```python
from build123d import *

# Parameters (mm, degrees)
SKETCH1_R           = 3
BOSS_EXTRUDE2_DEPTH = 12
SKETCH3_W           = 14.680148962
SKETCH3_H           = 3.5
CUT_EXTRUDE1_DEPTH  = 214.215717845
CUT_EXTRUDE4_DEPTH  = 6


with BuildPart() as part:
    # Sketch1 → Boss-Extrude2 (new body)
    with BuildSketch(Plane(origin=(0, 0, 0), x_dir=(1, 0, 0), z_dir=(0, 1, 0))):
        with BuildLine():
            ThreePointArc((49.32216584, -188.806160656), (56.59547157, -193.17640364), (60.965714553, -185.903097909))
            Line((60.965714554, -185.903097909), (16.76676248, -8.63078365))
            ThreePointArc((16.76676248, -8.63078365), (15.305067103, -5.385940236), (12.79956958, -2.858482163))
            Line((12.79956958, -2.858482163), (-5.735764363, 10.120098388))
            ThreePointArc((-5.735764363, 10.120098388), (-8.870108332, 13.694132698), (-10, 18.311618831))
            Line((-10, 18.311618831), (-10, 50.355948326))
            ThreePointArc((-10, 50.355948326), (-10.073223305, 50.532725021), (-10.25, 50.605948326))
            Line((-10.25, 50.605948326), (-11.322967039, 50.605948326))
            ThreePointArc((-11.322967039, 50.605948326), (-11.883595848, 50.434015556), (-12.251443729, 49.977339002))
            Line((-12.251443729, 49.977339002), (-13.876153382, 45.915564871))
            ThreePointArc((-13.876153382, 45.915564871), (-13.982191925, 45.601023533), (-14.052832331, 45.276692901))
            Line((-14.052832331, 45.276692901), (-19.445744306, 11.667622342))
            ThreePointArc((-19.445744306, 11.667622342), (-19.325125521, 8.055028023), (-17.928078586, 4.721314409))
            Line((-17.928078586, 4.721314409), (12.801336755, -42.329115693))
            Line((12.801336755, -42.329115693), (49.322165839, -188.806160656))
        make_face()
        with BuildLine():
            Line((53.747443969, -171.212996829), (57.618194299, -186.737728449))
            ThreePointArc((57.618194299, -186.737728449), (55.76084103, -189.828883385), (52.669686095, -187.971530117))
            Line((52.669686095, -187.971530117), (48.798935765, -172.446798496))
            ThreePointArc((48.798935765, -172.446798496), (50.656289033, -169.355643561), (53.747443969, -171.212996829))
        make_face(mode=Mode.SUBTRACT)
        with Locations(Location((0, 0, 0), (0, 0, 270))):
            Circle(SKETCH1_R, mode=Mode.SUBTRACT)
    extrude(amount=BOSS_EXTRUDE2_DEPTH)

    # Sketch3 → Cut-Extrude1 (cut, through all)
    with BuildSketch(Plane(origin=(-20.818600927, 0, -3.11186707), x_dir=(-0.15843335293481708, 0, 0.9873696737685596), z_dir=(-0.9873696737685597, 0, -0.1584333529348171))):
        Polygon((-42.704193729, 0), (-8.890997144, 0), (-22.384342691, 3.5), (-42.704193729, 3.5), align=None)
        Polygon((-22.384342691, 8.5), (-8.890997144, 12), (-42.704193729, 12), (-42.704193729, 8.5), align=None)
        with Locations((-50.04426821, 10.25)):
            Rectangle(SKETCH3_W, SKETCH3_H)
        with Locations((-50.04426821, 1.75)):
            Rectangle(SKETCH3_W, SKETCH3_H)
    extrude(amount=-CUT_EXTRUDE1_DEPTH, mode=Mode.SUBTRACT)

    # Sketch4 → Cut-Extrude4 (cut)
    with BuildSketch(Plane(origin=(0, 12, 0), x_dir=(1, 0, 0), z_dir=(0, 1, 0))):
        Polygon((-4.95077941, 9.570446006), (-17.928078586, 4.721314409), (8.620757021, -35.928145405), (10.712205441, -18.154940656), (16.76676248, -8.63078365), (17.432158169, -2.976226879), align=None)
    extrude(amount=-CUT_EXTRUDE4_DEPTH, mode=Mode.SUBTRACT)


solid = part.part
```
Design review of the part built by this model. Coordinates are the model's own, in mm. A direction names the side the tool comes from. Coordinates: 2 decimals unless noted, no trailing zeros. Order: outer loops, then holes, each group sorted by start corner. A loop starts at its lowest first (then second) coordinate and runs counter-clockwise, first axis right, second up.
1) Take a section at A-A, the plane x = 0. Give the boundary of the cut face in (y, z).
2) Clearance check with flat-ended pins moving along their axes: pin 1 (8 mm diameter, centred on x = -15, z = -39, fed in from -Y); pin 2 (2 mm diameter, centred on x = -14.5, z = -32, fed in from +Y); pin 3 (3 mm diameter, centred on y = 8, z = 94.5, fed in from +X). State where each tip first meets the part, or that it passes through.
3) Take a section at C-C, the plane z = 29. Give the boundary of the cut face in (x, y), and give its area (3 significant figures).
4) Wall thickness on line 1 along Z through (x, y) = (0, 3.95); line 2 along X through (y, z) = (6.5, 182.5); line 3 along Z through (x, y) = (0.5, 2): over which ranges is each line inside the solid? List them lowest first.
5) Take a section at B-B, the plane z = 0. Give the boundary of the cut face in (x, y), and give its area (3 significant figures).
6) Take a section at D-D, the plane x = 40.5. Give the boundary of the cut face in (y, z), and give its area (3 significant figures).
7) For faces 1 (the flat face through (-10, 6, -34)), 2 (the flat face through (55.656, 5.916, 178.867)), 3 (the flat face through (-11.3, 9, -7.2)), list the 3-axis set-ups (+Z, -Z, +X, -X, +Y, -Y) from which the entire face can be reached by the end or side of a thin tool; tool diameter is ignored.
8) Mouldability with a two-part tool opening along X and no side actions: class faces 4 (the flat face through (9.65, 9.04, 27.17)), 5 (the flat face through (50.76, 5.92, 180.32)), 6 (the flat face through (-1, 6, 8)) as +X half, -X half, draft (parallel to the pull), parting line (faces both ways), or undercut.
Returned:
1. outline: (0, -6.1) - (6, -6.1) - (6, -3) - (0, -3) - close; (0, 3) - (6, 3) - (6, 22.73) - (0, 22.73) - close
2. pin 1: stops at y = 3.5
2. pin 2: stops at y = 8.5
2. pin 3: stops at x = 38.55
3. outline: (4.1, 0) - (21.85, 0) - (21.85, 12) - (9.44, 12) - (9.44, 6) - (4.1, 6) - close
3. area: 181 mm2
4. line 1: z = -6.1 to -3, 3 to 22.73
4. line 2: x = 47.75 to 51.31, 56.56 to 60.12
4. line 3: z = -5.75 to -2.96, 2.96 to 23.49
5. outline: (-14.84, 0) - (-3, 0) - (-3, 6) - (-14.84, 6) - close; (3, 0) - (8.72, 0) - (8.72, 6) - (3, 6) - close
5. area: 105 mm2
6. outline: (0, 103.82) - (12, 103.82) - (12, 153.42) - (0, 153.42) - close
6. area: 595 mm2
7. face 1: -Z, +X, +Y, -Y
7. face 2: +Y, -Y
7. face 3: +Z, +X, +Y
8. face 4: -X half
8. face 5: undercut
8. face 6: draft
